from build123d import *

# Parameters (mm, degrees)
F0_W     = 80
F0_H     = 12.5
F1_DEPTH = 3
F2_R     = 5
F4_D     = 5


with BuildPart() as f1:
    # F0 (on Top) → F1 (new body)
    with BuildSketch(Plane.XY):
        Rectangle(F0_W, F0_H)
    extrude(amount=F1_DEPTH)

    # F2
    f2_edges = [f1.edges().sort_by_distance(p)[0] for p in [
        (40, -6.25, 1.5),
        (40, 6.25, 1.5),
        (-40, -6.25, 1.5),
        (-40, 6.25, 1.5),
    ]]
    fillet(f2_edges, radius=F2_R)

    # F4 (through all)
    with Locations(Plane(origin=(0, 0, 0), x_dir=(1, 0, 0), z_dir=(0, 0, -1))):
        with Locations((-35, 0), (0, 0), (35, 0)):
            Hole(F4_D / 2)


solid = f1.part
Geometry: final body of the model. Coordinates: model frame, mm. Round coordinates to 2 decimals unless told otherwise and drop trailing zeros. Loops run counter-clockwise (first coordinate to the right, second up) from the corner with the lowest first, then second, coordinate; pieces in that order, holes last.
Q1. Pull-direction query (X, two-part tool) for faces 1 (the flat face through (-1, 3, 3)), 2 (the cylindrical face through (-37.31, 0.96, 1.52)), 3 (the cylindrical face through (-38.57, 4.75, 1.52)), 4 (the cylindrical face through (32.69, 0.96, 1.52)); classes: released by +X, released by -X, zero draft, split by the parting line, or undercut.
Q2. Pin query (flat end, axial travel): P1, Ø4, axis at x = 0, y = 0, coming from the -Z side. Return the tip coordinate at first contact, or that it passes through.
Q3. Material intervals for L1, parallel to X at y = -0.25, z = 1.3; L2, parallel to X at y = -1.5, z = 2.75; L3, parallel to Y at x = -35, z = 1.6, sorted ascending.
Q4. Section D-D on y = -4.25. Return loops of the section in (x, z), plus the area to 3 significant figures.
Q5. Section B-B on z = 2.35. Return loops of the section in (x, y).
Q6. Section A-A on y = 0. Return loops of the section in (x, z).
Q7. Section C-C on x = 0. Return loops of the section in (y, z), plus the area to 3 significant figures.
Evaluation:
1. face 1: zero draft
1. face 2: undercut
1. face 3: released by -X
1. face 4: undercut
2. P1: passes through
3. L1: x = -40 to -37.49, -32.51 to -2.49, 2.49 to 32.51, 37.49 to 40
3. L2: x = -39.99 to -37, -33 to -2, 2 to 33, 37 to 39.99
3. L3: y = -6.25 to -2.5, 2.5 to 6.25
4. outline: (-39, 0) - (39, 0) - (39, 3) - (-39, 3) - close
4. area: 234 mm2
5. outline: (-40, -1.25) arc R5 ccw to (-35, -6.25) - (35, -6.25) arc R5 ccw to (40, -1.25) - (40, 1.25) arc R5 ccw to (35, 6.25) - (-35, 6.25) arc R5 ccw to (-40, 1.25) - close; hole circle Ø5 at (-35, 0); hole circle Ø5 at (0, 0); hole circle Ø5 at (35, 0)
6. outline: (-40, 0) - (-37.5, 0) - (-37.5, 3) - (-40, 3) - close; (-32.5, 0) - (-2.5, 0) - (-2.5, 3) - (-32.5, 3) - close; (2.5, 0) - (32.5, 0) - (32.5, 3) - (2.5, 3) - close; (37.5, 0) - (40, 0) - (40, 3) - (37.5, 3) - close
7. outline: (-6.25, 0) - (-2.5, 0) - (-2.5, 3) - (-6.25, 3) - close; (2.5, 0) - (6.25, 0) - (6.25, 3) - (2.5, 3) - close
7. area: 22.5 mm2
